```python
from build123d import *

# Parameters (mm, degrees)
F0_W     = 42.2
F0_H     = 55
F1_DEPTH = 2
F2_R     = 3


with BuildPart() as f1:
    # F0 (on Top) → F1 (new body)
    with BuildSketch(Plane.XY):
        with Locations((21.1, 27.5)):
            Rectangle(F0_W, F0_H)
        with BuildLine():
            ThreePointArc((11.625, 6.7573734957), (8.6170854504, 5.9040433436), (10.7287878788, 8.2097829516))
            ThreePointArc((10.7287878788, 8.2097829516), (11.3829145496, 7.6107036478), (11.625, 6.7573734957))
        make_face(mode=Mode.SUBTRACT)
        with BuildLine():
            Line((7.225, 44.3786867478), (28.8775671832, 44.3786867478))
            Line((28.8775671832, 44.3786867478), (34.975, 44.3786867478))
            ThreePointArc((34.975, 44.3786867478), (36.6, 46.0036867478), (38.225, 44.3786867478))
            ThreePointArc((38.225, 44.3786867478), (37.7490485194, 43.2296382284), (36.6, 42.7536867478))
            Line((36.6, 42.7536867478), (36.6, 15.0036867478))
            ThreePointArc((36.6, 15.0036867478), (37.7490485194, 14.5277352673), (38.225, 13.3786867478))
            ThreePointArc((38.225, 13.3786867478), (36.6, 11.7536867478), (34.975, 13.3786867478))
            Line((34.975, 13.3786867478), (13.3224328168, 13.3786867478))
            Line((13.3224328168, 13.3786867478), (7.225, 13.3786867478))
            ThreePointArc((7.225, 13.3786867478), (4.4509514806, 12.2296382284), (5.6, 15.0036867478))
            Line((5.6, 15.0036867478), (5.6, 42.7536867478))
            ThreePointArc((5.6, 42.7536867478), (4.4509514806, 45.5277352673), (7.225, 44.3786867478))
        make_face(mode=Mode.SUBTRACT)
        with BuildLine():
            ThreePointArc((31.4712121212, 49.5475905441), (31.3466698479, 52.3829145496), (33.825, 51))
            ThreePointArc((33.825, 51), (33.0533301521, 49.6170854504), (31.4712121212, 49.5475905441))
        make_face(mode=Mode.SUBTRACT)
        with BuildLine():
            Line((26.1454545455, 38.9338291352), (28.8775671832, 44.3786867478))
            Line((28.8775671832, 44.3786867478), (7.225, 44.3786867478))
            ThreePointArc((7.225, 44.3786867478), (6.7490485194, 43.2296382284), (5.6, 42.7536867478))
            Line((5.6, 42.7536867478), (5.6, 15.0036867478))
            ThreePointArc((5.6, 15.0036867478), (6.7490485194, 14.5277352673), (7.225, 13.3786867478))
            Line((7.225, 13.3786867478), (13.3224328168, 13.3786867478))
            Line((13.3224328168, 13.3786867478), (16.0545454545, 18.8235443605))
            ThreePointArc((16.0545454545, 18.8235443605), (11.0448576127, 33.9241412933), (26.1454545455, 38.9338291352))
        make_face()
        with BuildLine():
            Line((34.975, 44.3786867478), (28.8775671832, 44.3786867478))
            Line((28.8775671832, 44.3786867478), (26.1454545455, 38.9338291352))
            ThreePointArc((26.1454545455, 38.9338291352), (30.674023805, 34.7863570316), (32.35, 28.8786867478))
            ThreePointArc((32.35, 28.8786867478), (27.0076702838, 19.3046629429), (16.0545454545, 18.8235443605))
            Line((16.0545454545, 18.8235443605), (13.3224328168, 13.3786867478))
            Line((13.3224328168, 13.3786867478), (34.975, 13.3786867478))
            ThreePointArc((34.975, 13.3786867478), (35.4509514806, 14.5277352673), (36.6, 15.0036867478))
            Line((36.6, 15.0036867478), (36.6, 42.7536867478))
            ThreePointArc((36.6, 42.7536867478), (35.4509514806, 43.2296382284), (34.975, 44.3786867478))
        make_face()
    extrude(amount=F1_DEPTH)

    # F2
    f2_edges = [f1.edges().sort_by_distance(p)[0] for p in [
        (42.2, 55, 1),
        (0, 55, 1),
        (0, 0, 1),
        (42.2, 0, 1),
    ]]
    fillet(f2_edges, radius=F2_R)


solid = f1.part
```
Work out the finished part from the listing and answer in its coordinate system (mm). Give positions to 0.01 mm unless a question says otherwise; leave off trailing zeros. Loops run counter-clockwise (first coordinate to the right, second up) from the corner with the lowest first, then second, coordinate; pieces in that order, holes last. Notation, with made-up numbers: (-15.5, -33) - (12.5, -33) arc R27 cw to (12.5, -4) - close; hole circle Ø7 at (-23.75, 70.25). An arc over 180 degrees is marked (long way). Use CSV: the item, a comma, the result in double quotes. Start each with the question number.
(1) Find the intervals of material crossed by L1, parallel to Y at x = 5.6, z = 1; L2, parallel to X at y = 13.5, z = 0.85; L3, parallel to X at y = 51, z = 0.8 (3 decimals), in increasing order.
(2) Find section C-C, the plane y = 27. Determine the outline of the cut face in (x, z).
(3) Find section A-A, the plane z = 0.55. Determine the outline of the cut face in (x, y) (3 decimals).
(4) Find section B-B, the plane x = 30. Determine the outline of the cut face in (y, z), plus the area to 3 significant figures.
(5) This flat-tipped pin is pushed along its axis until it touches: pin 1 (12 mm diameter, centred on x = 18.5, y = 34.5, fed in from +Z). Where does it stop, or does it pass through?
Results found:
1,L1,"0 to 11.75, 15 to 42.75, 46 to 55"
1,L2,"0 to 3.98, 7.22 to 34.98, 38.22 to 42.2"
1,L3,"0 to 30.575, 33.825 to 42.2"
2,outline,"(0, 0) - (10.01, 0) - (10.01, 2) - (0, 2) - close; (32.19, 0) - (42.2, 0) - (42.2, 2) - (32.19, 2) - close"
3,outline,"(0, 3) arc R3 ccw to (3, 0) - (39.2, 0) arc R3 ccw to (42.2, 3) - (42.2, 52) arc R3 ccw to (39.2, 55) - (3, 55) arc R3 ccw to (0, 52) - close; hole circle Ø3.25 at (5.6, 13.379); hole circle Ø3.25 at (5.6, 44.379); hole circle Ø3.25 at (10, 6.757); hole circle Ø22.5 at (21.1, 28.879); hole circle Ø3.25 at (32.2, 51); hole circle Ø3.25 at (36.6, 13.379); hole circle Ø3.25 at (36.6, 44.379)"
4,outline,"(0, 0) - (22, 0) - (22, 2) - (0, 2) - close; (35.76, 0) - (55, 0) - (55, 2) - (35.76, 2) - close"
4,area,"82.5 mm^2"
5,pin 1,"z = 2"
